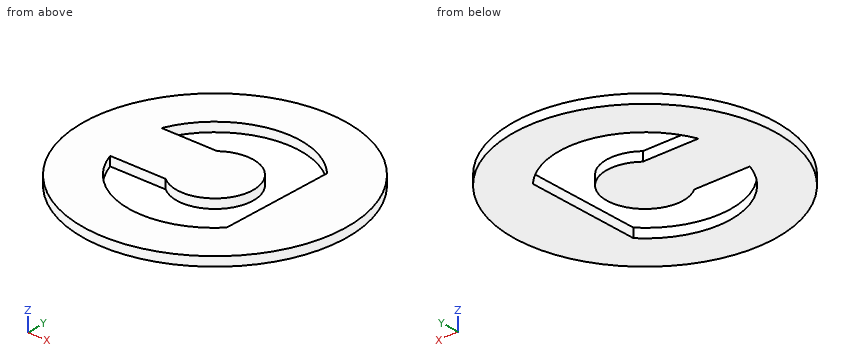
```python
from build123d import *

# Parameters (mm, degrees)
F0_R     = 36.5125
F1_DEPTH = 2.54


with BuildPart() as f1:
    # F0 (on Top) → F1 (new body)
    with BuildSketch(Plane.XY):
        with Locations((2.223555, 0)):
            Circle(F0_R)
        with BuildLine():
            Line((19.686055, 16.189387), (19.686055, -16.189387))
            ThreePointArc((19.686055, -16.189387), (-2.415954, -23.356158), (-20.100791, -8.286056))
            Line((-20.100791, -8.286056), (-4.414684, -8.286056))
            ThreePointArc((-4.414684, -8.286056), (12.840755, 0), (-4.414684, 8.286056))
            Line((-4.414684, 8.286056), (-20.100791, 8.286056))
            ThreePointArc((-20.100791, 8.286056), (-2.415954, 23.356158), (19.686055, 16.189387))
        make_face(mode=Mode.SUBTRACT)
    extrude(amount=F1_DEPTH)


solid = f1.part
```
Read the model definition and answer for the solid it produces. Units are mm, in the model's axes. Coordinates: 2 decimals unless noted, no trailing zeros. Order: outer loops, then holes, each group sorted by start corner. A loop starts at its lowest first (then second) coordinate and runs counter-clockwise, first axis right, second up. Notation, with made-up numbers: (-33.75, -28) - (18.25, -28) arc R22 ccw to (18.25, 0) - close; hole circle Ø11 at (68.25, -20). An arc over 180 degrees is marked (long way). Answer as a JSON object with one key per item and string values. Group by question number.
Item 1: Section D-D (x = -16) is taken. Give the vertices of the cut face in (y, z).
Item 2: Section A-A (y = 0) is taken. Give the vertices of the cut face in (x, z), plus the area to 3 significant figures.
Item 3: Section B-B (x = 14.5) is taken. Give the vertices of the cut face in (y, z), plus the area to 3 significant figures.
Item 4: Flat-ended cylindrical pins translate along their axes: P1, Ø1, axis at x = -14, z = 0.5, coming from the +Y side; P2, Ø1.3, axis at x = -12, z = 1, coming from the +Y side; P3, Ø10, axis at x = -1.5, y = 20.5, coming from the -Z side; P4, Ø1.5, axis at y = -25, z = 0.5, coming from the +X side. Find the tip coordinate at first contact, or state that the pin passes through.
Item 5: Section C-C (z = 1.3) is taken. Give the vertices of the cut face in (x, y) (1 decimal).
Item 6: Consider probe 1 along Y at (x, z) = (2, 2.15); probe 2 along X at (y, z) = (-9.5, 0.9); probe 3 along Y at (x, z) = (-12, 2.1). Determine where each line is inside the solid, lowest interval first. Write a range as from..to.
Results are:
{
 "1": {"outline": "(-31.64, 0) - (-15.33, 0) - (-15.33, 2.54) - (-31.64, 2.54) - close; (-8.29, 0) - (8.29, 0) - (8.29, 2.54) - (-8.29, 2.54) - close; (15.33, 0) - (31.64, 0) - (31.64, 2.54) - (15.33, 2.54) - close"},
 "2": {"outline": "(-34.29, 0) - (12.84, 0) - (12.84, 2.54) - (-34.29, 2.54) - close; (19.69, 0) - (38.74, 0) - (38.74, 2.54) - (19.69, 2.54) - close", "area": "168 mm^2"},
 "3": {"outline": "(-34.39, 0) - (-20.4, 0) - (-20.4, 2.54) - (-34.39, 2.54) - close; (20.4, 0) - (34.39, 0) - (34.39, 2.54) - (20.4, 2.54) - close", "area": "71.0 mm^2"},
 "4": {"P1": "stops at y = 32.95", "P2": "stops at y = 33.9", "P3": "stops at z = 0", "P4": "stops at x = 29.52"},
 "5": {"outline": "circle Ø73 at (2.2, 0); hole (-20.1, -8.3) arc R23.8 ccw to (19.7, -16.2) - (19.7, 16.2) arc R23.8 ccw to (-20.1, 8.3) - (-4.4, 8.3) arc R10.6 cw (long way) to (-4.4, -8.3) - close"},
 "6": {"probe 1": "y = -36.51..-23.81, -10.61..10.61, 23.81..36.51", "probe 2": "x = -33.03..-19.61, -2.52..6.96, 19.69..37.48", "probe 3": "y = -33.63..-19.1, -8.29..8.29, 19.1..33.63"}
}
